Answer from the drawing. Dimensions are ordinates in mm from the lowest x, y and z of the part. A direction names the side the tool comes from. Give positions to 0.01 mm unless a question says otherwise; leave off trailing zeros. Write each loop counter-clockwise with the first axis right and the second up, starting at its lowest first coordinate (ties: lowest second). Pieces come first, ordered by that corner, then holes. Notation, with made-up numbers: (33, -4) -> (92, -4) arc R18 cw to (92, 0) -> close; hole circle Ø8 at (3, 81). An arc over 180 degrees is marked (long way). Write item = value, one per line.
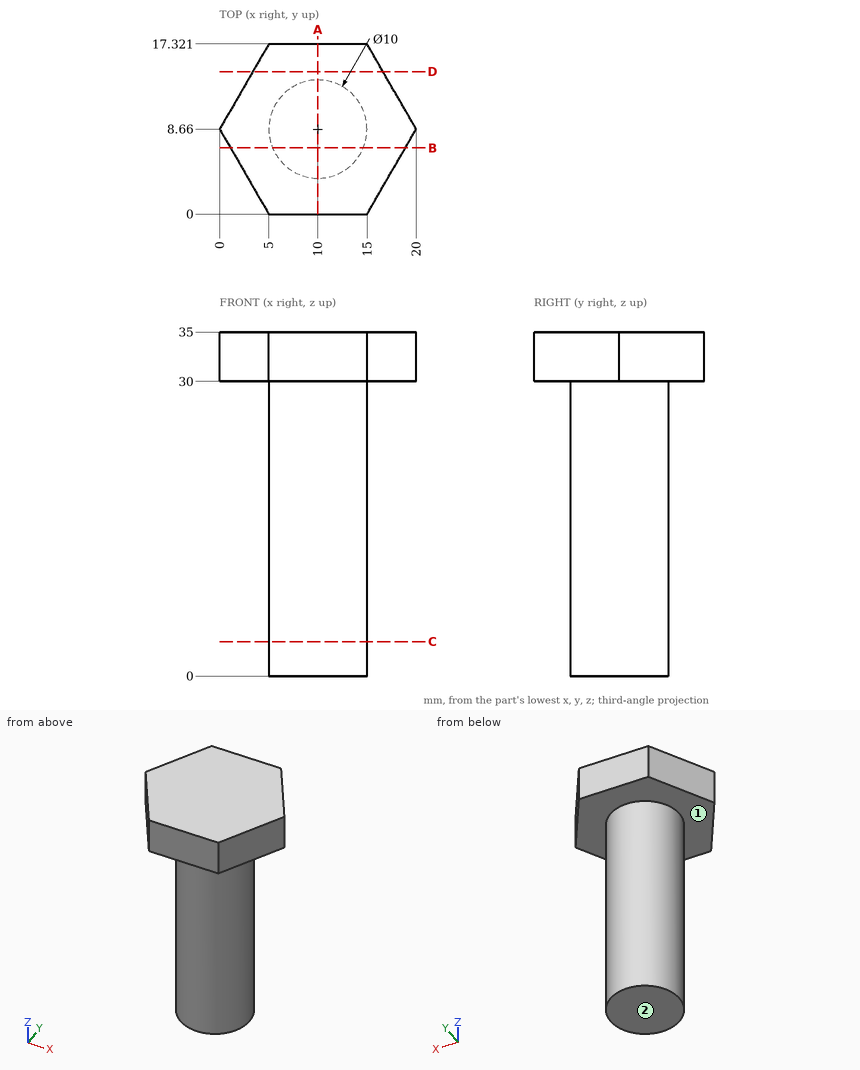
(1) Given P1, Ø3, axis at y = 8, z = 26, coming from the +X side; P2, Ø5, axis at y = 14, z = 18, coming from the -X side (1 decimal); P3, Ø6, axis at x = 10.5, z = 24.5, coming from the -Y side, each flat-ended and moving along its own axis, determine where each tip first touches the part or whether it passes through.
Checks:
P1 = 15
P2 = 5.9
P3 = 3.66
(2) A tool of negligible diameter and unlimited length cuts with its end or side. For the marked faces 1 and 2, from which of +Z, -Z, +X, -X, +Y, -Y can it reach the whole face along a straight path? Write none if from no direction.
Checks:
face_1 = -Z
face_2 = -Z, +X, -X, +Y, -Y
(3) Consider L1, parallel to Z at x = 9.5, y = 14; L2, parallel to X at y = 6.25, z = 3.5; L3, parallel to X at y = 4.75, z = 31.5. Determine where each line is inside the solid, lowest interval first.
Checks:
L1 = 30 to 35
L2 = 5.62 to 14.38
L3 = 2.26 to 17.74
(4) The part is cut by section C-C on z = 3.5. Determine the outline of the cut face in (x, y).
Checks:
outline = circle Ø10 at (10, 8.66)
(5) The part is cut by section B-B on y = 6.75. Determine the outline of the cut face in (x, z), plus the area to 3 significant figures.
Checks:
outline = (1.1, 30) -> (5.38, 30) -> (5.38, 0) -> (14.62, 0) -> (14.62, 30) -> (18.9, 30) -> (18.9, 35) -> (1.1, 35) -> close
area = 366 mm²
(6) The part is cut by section D-D on y = 14.5. Determine the outline of the cut face in (x, z).
Checks:
outline = (3.37, 30) -> (16.63, 30) -> (16.63, 35) -> (3.37, 35) -> close
(7) The part is cut by section A-A on x = 10. Determine the outline of the cut face in (y, z).
Checks:
outline = (0, 30) -> (3.66, 30) -> (3.66, 0) -> (13.66, 0) -> (13.66, 30) -> (17.32, 30) -> (17.32, 35) -> (0, 35) -> close
